Part model, mm, in its own coordinate system. Face numbers are marked on the shaded views. A direction names the side the tool comes from. Coordinates: 2 decimals unless noted, no trailing zeros. Loops run counter-clockwise (first coordinate to the right, second up) from the corner with the lowest first, then second, coordinate; pieces in that order, holes last. Notation, with made-up numbers: M 55.25,58.5 L 74.25,58.5 A14 ccw 74.25,78.5 Z; hole C 41.5,49 d2. An arc over 180 degrees is marked long. Use a Markdown table: item, result. Add a question column.
1) Pin check, flat tips, straight feed: pin 1 Ø11 at (x, z) = (0, 0) entering from +Y; pin 2 Ø2 at (x, z) = (17, -13) entering from +Y; pin 3 Ø5 at (x, z) = (-16, -2) entering from -Y; pin 4 Ø1.3 at (x, y) = (19.5, 2.5) entering from +Z. Stop position of each tip, or through.
2) Band-saw the part on D-D (z = 10). List the corners of the cut face in (x, y), plus the area to 3 significant figures.
3) Wall check: probe 1 along X at (y, z) = (5, 0); probe 2 along X at (y, z) = (18.5, 0); probe 3 along Z at (x, y) = (3, 5). Give the ranges that are in metal, low to high. Write a range as from..to.
4) Band-saw the part on A-A (y = 2.5). List the corners of the cut face in (x, z).
5) Tool access for the marked faces 5 and 6: list every direction of +Z, -Z, +X, -X, +Y, -Y with a clear straight run to the whole face (end or side of a thin tool).
6) Band-saw the part on C-C (y = 17). List the corners of the cut face in (x, z), plus the area to 3 significant figures.
7) Band-saw the part on B-B (x = 16.5). List the corners of the cut face in (y, z).
8) Pull direction X, two halves, no side cores. Call the marked faces 1, 2, 3 and 4: released by +X, released by -X, zero draft, split by the parting line, or undercut.
from build123d import *
from build123d.topology import SkipClean

# Parameters (mm, degrees)
ESQUISSE2_R                  = 9
BOSS_EXTRU_1_DEPTH           = 22
ESQUISSE5_R                  = 5
BOSS_EXTRU_3_DEPTH           = 2
ESQUISSE6_R                  = 6
ENL_V_MAT_EXTRU_2_DEPTH      = 14
ESQUISSE7_R                  = 4
ENL_V_MAT_EXTRU_3_DEPTH      = 19.920887928
ESQUISSE8_R                  = 5
ENL_V_MAT_EXTRU_4_DEPTH      = 0.7
ENL_V_START                  = -0.7
ESQUISSE9_R                  = 5
ENL_V_MAT_EXTRU_5_DEPTH      = 0.7
BOSS_EXTRU_4_START           = 2
ESQUISSE11_R                 = 9
ESQUISSE11_R_2               = 5
BOSS_EXTRU_4_DEPTH           = 2
BOSS_EXTRU_5_DEPTH           = 2
R_P_TITION_CIRCULAIRE1_COUNT = 3
BOSS_EXTRU_6_DEPTH           = 6.5
R_P_TITION_CIRCULAIRE2_COUNT = 3
D_GAGEMENT_M51_D             = 5.5
D_GAGEMENT_M51_CSINK_D       = 5.55
D_GAGEMENT_M51_CSINK_ANGLE   = 90
R_P_TITION_CIRCULAIRE3_COUNT = 3
CONG_1_R                     = 3
CONG_2_R                     = 3
CONG_3_R                     = 2


with BuildPart() as part:
    # Esquisse2 → Boss.-Extru.1 (new body)
    with BuildSketch(Plane(origin=(0, 0, 0), x_dir=(1, 0, 0), z_dir=(0, 1, 0))):
        with Locations(Location((0, 0, 0), (0, 0, 270))):
            Circle(ESQUISSE2_R)
    extrude(amount=BOSS_EXTRU_1_DEPTH)

    # Esquisse5 → Boss.-Extru.3 (add)
    with BuildSketch(Plane(origin=(0, 22, 0), x_dir=(1, 0, 0), z_dir=(0, 1, 0))):
        Circle(ESQUISSE5_R)
    extrude(amount=-BOSS_EXTRU_3_DEPTH)

    # Esquisse6 → Enl_v. mat.-Extru.2 (cut)
    with BuildSketch(Plane(origin=(0, 22, 0), x_dir=(1, 0, 0), z_dir=(0, 1, 0))):
        with Locations(Location((0, 0, 0), (0, 0, 270))):
            Circle(ESQUISSE6_R)
    extrude(amount=-ENL_V_MAT_EXTRU_2_DEPTH, mode=Mode.SUBTRACT)

    # Esquisse7 → Enl_v. mat.-Extru.3 (cut, through all)
    with BuildSketch(Plane(origin=(0, 8, 0), x_dir=(1, 0, 0), z_dir=(0, 1, 0))):
        with Locations(Location((0, 0, 0), (0, 0, 270))):
            Circle(ESQUISSE7_R)
    extrude(amount=-ENL_V_MAT_EXTRU_3_DEPTH, mode=Mode.SUBTRACT)

    # Esquisse8 → Enl_v. mat.-Extru.4 (cut)
    with BuildSketch(Plane.XZ):
        with Locations(Location((0, 0, 0), (0, 0, 270))):
            Circle(ESQUISSE8_R)
    extrude(amount=-ENL_V_MAT_EXTRU_4_DEPTH, mode=Mode.SUBTRACT)

    # Esquisse9 → Enl_v. mat.-Extru.5 (cut)
    with BuildSketch(Plane(origin=(0, 8, 0), x_dir=(1, 0, 0), z_dir=(0, 1, 0)).offset(ENL_V_START)):
        with Locations(Location((0, 0, 0), (0, 0, 90))):
            Circle(ESQUISSE9_R)
    extrude(amount=ENL_V_MAT_EXTRU_5_DEPTH, mode=Mode.SUBTRACT)

    # Esquisse11 → Boss.-Extru.4 (add)
    with BuildSketch(Plane.XZ.offset(BOSS_EXTRU_4_START)):
        with Locations(Location((0, 0, 0), (0, 0, 270))):
            Circle(ESQUISSE11_R)
        with Locations(Location((0, 0, 0), (0, 0, 270))):
            Circle(ESQUISSE11_R_2, mode=Mode.SUBTRACT)
    extrude(amount=-BOSS_EXTRU_4_DEPTH)

    # Esquisse12 → Boss.-Extru.5 (add)
    with SkipClean():  # the faces are left unmerged after this step: merging them gives an invalid solid
        with BuildSketch(Plane.XZ.offset(2)):
            with BuildLine():
                Line((-4.8, 2.012544091), (-4.8, 28.05))
                Line((-4.8, 28.05), (5, 28.05))
                Line((5, 28.05), (5, 1.445798644))
                ThreePointArc((5, 1.445798644), (0.300499751, 5.196155658), (-4.8, 2.012544091))
            make_face()
        boss_extru_5 = extrude(amount=-BOSS_EXTRU_5_DEPTH)

    # R_p_tition circulaire1: Boss.-Extru.5 ×3 about axis
    with SkipClean():  # the faces are left unmerged after this step: merging them gives an invalid solid
        r_p_tition_circulaire1_axis = Axis((0, 0, 0), (0, 1, 0))
        for i in range(1, R_P_TITION_CIRCULAIRE1_COUNT):
            add(boss_extru_5.rotate(r_p_tition_circulaire1_axis, i * 360 / R_P_TITION_CIRCULAIRE1_COUNT))

    # Esquisse13 → Boss.-Extru.6 (add)
    with SkipClean():  # the faces are left unmerged after this step: merging them gives an invalid solid
        with BuildSketch(Plane.XZ.offset(2)):
            Polygon((-2.35, 28.05), (-4.8, 23.806475521), (-2.35, 19.562951043), (2.55, 19.562951043), (5, 23.806475521), (2.55, 28.05), align=None)
        boss_extru_6 = extrude(amount=-BOSS_EXTRU_6_DEPTH)

    # R_p_tition circulaire2: Boss.-Extru.6 ×3 about axis
    with SkipClean():  # the faces are left unmerged after this step: merging them gives an invalid solid
        r_p_tition_circulaire2_axis = Axis((0, 0, 0), (0, 1, 0))
        for i in range(1, R_P_TITION_CIRCULAIRE2_COUNT):
            add(boss_extru_6.rotate(r_p_tition_circulaire2_axis, i * 360 / R_P_TITION_CIRCULAIRE2_COUNT))

    # D_gagement M51 (through all)
    with Locations(Plane(origin=(0, 4.5, 0), x_dir=(1, 0, 0), z_dir=(0, 1, 0))):
        with Locations((0.1, -23.806475521)):
            d_gagement_m51 = CounterSinkHole(D_GAGEMENT_M51_D / 2, D_GAGEMENT_M51_CSINK_D / 2, counter_sink_angle=D_GAGEMENT_M51_CSINK_ANGLE)

    # R_p_tition circulaire3: D_gagement M51 ×3 about axis
    with SkipClean():  # the faces are left unmerged after this step: merging them gives an invalid solid
        r_p_tition_circulaire3_axis = Axis((0, 0, 0), (0, 1, 0))
        for i in range(1, R_P_TITION_CIRCULAIRE3_COUNT):
            add(d_gagement_m51.rotate(r_p_tition_circulaire3_axis, i * 360 / R_P_TITION_CIRCULAIRE3_COUNT), mode=Mode.SUBTRACT)

    # Cong_1
    cong_1_edges = [part.edges().sort_by_distance(p)[0] for p in [
        (-4.8, -1, 7.613146524),
    ]]
    fillet(cong_1_edges, radius=CONG_1_R)

    # Cong_2
    # the kernel refuses this fillet: 3 mm, written as the material it adds along each edge
    with BuildSketch(Plane(origin=(5, 0, 7.483314774), x_dir=(0, 0, 1), z_dir=(0, -1, 0)), Plane(origin=(3.980740698, 0, -8.071784406), x_dir=(0.8660254037844388, 0, -0.4999999999999996), z_dir=(0, -1, 0)), Plane(origin=(-8.980740698, 0, 0.588469632), x_dir=(-0.8660254037844384, 0, -0.5000000000000007), z_dir=(0, -1, 0))) as cong_2_piece_1:
        with BuildLine():
            CenterArc((1.460957136, -3), CONG_2_R, 90, 48.189685104)
            ThreePointArc((-0.775110841, -1), (-0.369961078, -0.513637566), (0, 0))
            Line((0, 0), (1.460957136, 0))
        make_face()
    extrude(amount=2)
    with BuildSketch(Plane(origin=(8.993178293, 0, 0.350348676), x_dir=(0.866025403784439, 0, -0.49999999999999933), z_dir=(0, -1, 0)), Plane(origin=(-4.193178293, 0, -7.9634952), x_dir=(-0.8660254037844389, 0, -0.4999999999999995), z_dir=(0, -1, 0))) as cong_2_piece_2:
        with BuildLine():
            CenterArc((1.506063968, 3), CONG_2_R, 220.541601874, 49.458398126)
            ThreePointArc((-0.773738655, 1.05), (-0.367823404, 0.539034826), (0, 0))
            Line((0, 0), (1.506063968, 0))
        make_face()
    extrude(amount=2)

    # Cong_3
    cong_3_edges = [part.edges().sort_by_distance(p)[0] for p in [
        (5, -1, 28.05),
        (-4.8, -1, 28.05),
        (21.792012576, -1, -18.355127019),
        (-26.792012576, -1, -9.694872981),
        (26.692012576, -1, -9.868078062),
        (-21.892012576, -1, -18.181921938),
    ]]
    fillet(cong_3_edges, radius=CONG_3_R)


solid = part.part
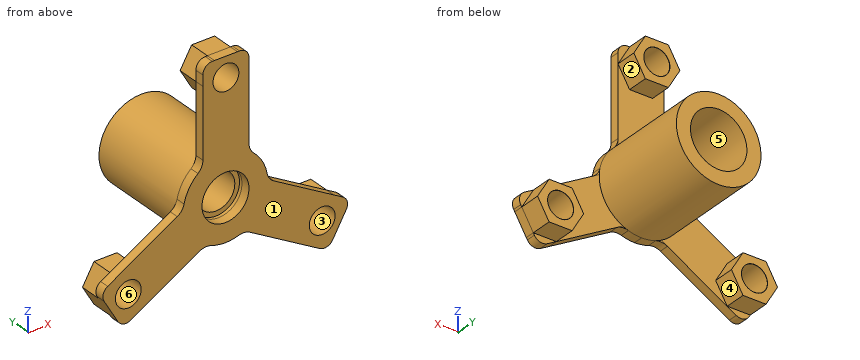
Entries:
| question | item | result |
|---|---|---|
| 1 | pin 1 | y = 8 |
| 1 | pin 2 | y = 4.5 |
| 1 | pin 3 | y = -2 |
| 1 | pin 4 | z = -7.75 |
| 2 | outline | M -4.8,-2 L 5,-2 L 5,0 L -4.8,0 Z |
| 2 | area | 19.6 mm2 |
| 3 | probe 1 | -9..-4, 4..9 |
| 3 | probe 2 | -9..-6, 6..9 |
| 3 | probe 3 | -8.49..-2.65, 2.65..8.49 |
| 4 | outline | M -25.57,-11.82 L -23.12,-16.06 L -18.22,-16.06 L -15.77,-11.82 L -18.22,-7.57 L -23.12,-7.57 Z; C 0,0 d18; M -4.8,23.81 L -2.35,19.56 L 2.55,19.56 L 5,23.81 L 2.55,28.05 L -2.35,28.05 Z; M 15.67,-11.99 L 18.12,-16.23 L 23.02,-16.23 L 25.47,-11.99 L 23.02,-7.75 L 18.12,-7.75 Z; hole C -20.67,-11.82 d5.5; hole C 0,0 d8; hole C 0.1,23.81 d5.5; hole C 20.57,-11.99 d5.5 |
| 5 | face 5 | +Y |
| 5 | face 6 | +Y, -Y |
| 6 | outline | C 0,0 d18; hole C 0,0 d12 |
| 6 | area | 141 mm2 |
| 7 | outline | M -2,-15.3 L 0,-15.3 L 0,-13.43 L 4.5,-13.43 L 4.5,-10.55 L 0,-10.55 L 0,-3.98 L -2,-3.98 Z |
| 8 | face 1 | zero draft |
| 8 | face 2 | released by +X |
| 8 | face 3 | undercut |
| 8 | face 4 | undercut |
